```python
from build123d import *

# Parameters (mm, degrees)
SKETCH1_W                                            = 106.5
SKETCH1_H                                            = 26
BOSS_EXTRUDE1_DEPTH                                  = 8
CUT_EXTRUDE1_START                                   = -26
CUT_EXTRUDE1_OUTLINE_W                               = 6
CUT_EXTRUDE1_OUTLINE_H                               = 6.5
CUT_EXTRUDE1_OUTLINE_W_2                             = 0.5
CUT_EXTRUDE1_OUTLINE_H_2                             = 7.5
CUT_EXTRUDE1_DEPTH                                   = 26
FILLET1_R                                            = 0.5
CSK_FOR_M1_6_COUNTERSUNK_FLAT_HEAD_SCREW_D           = 1.8
CSK_FOR_M1_6_COUNTERSUNK_FLAT_HEAD_SCREW_DEPTH       = 15
CSK_FOR_M1_6_COUNTERSUNK_FLAT_HEAD_SCREW_CSINK_D     = 3.6
CSK_FOR_M1_6_COUNTERSUNK_FLAT_HEAD_SCREW_CSINK_ANGLE = 90
CSK_FOR_M1_6_COUNTERSUNK_FLAT_HEAD_SCREW_TIP         = 0.540774557
SKETCH14_W                                           = 97
SKETCH14_H                                           = 24
CUT_EXTRUDE7_DEPTH                                   = 110.919288571
SKETCH14_3_W                                         = 97
SKETCH14_3_H                                         = 24
BOSS_EXTRUDE3_DEPTH                                  = 1
SKETCH18_W                                           = 97
SKETCH18_H                                           = 24
CUT_EXTRUDE8_DEPTH                                   = 10
SKETCH20_W                                           = 97
SKETCH20_H                                           = 24
SKETCH20_W_2                                         = 93
SKETCH20_H_2                                         = 20
BOSS_EXTRUDE4_DEPTH                                  = 8
SKETCH20_2_W                                         = 97
SKETCH20_2_H                                         = 24
SKETCH20_2_W_2                                       = 93
SKETCH20_2_H_2                                       = 20
CUT_EXTRUDE9_DEPTH                                   = 1.5


# Read off the part's stored shape, not the designer's step: Cut-Extrude1
with BuildPart() as part:
    # Sketch1 → Boss-Extrude1 (new body)
    with BuildSketch(Plane(origin=(0, 0, 0), x_dir=(1, 0, 0), z_dir=(0, 1, 0))):
        with Locations((53.25, -13)):
            Rectangle(SKETCH1_W, SKETCH1_H)
    extrude(amount=BOSS_EXTRUDE1_DEPTH)

    # Cut-Extrude1 outline → Cut-Extrude1 (cut)
    with BuildSketch(Plane.XY.offset(26).offset(CUT_EXTRUDE1_START)):
        with Locations((3, 4.75)):
            Rectangle(CUT_EXTRUDE1_OUTLINE_W, CUT_EXTRUDE1_OUTLINE_H)
        with Locations((106.25, 4.25)):
            Rectangle(CUT_EXTRUDE1_OUTLINE_W_2, CUT_EXTRUDE1_OUTLINE_H_2)
    extrude(amount=CUT_EXTRUDE1_DEPTH, mode=Mode.SUBTRACT)

    # Fillet1
    fillet1_edges = [part.edges().sort_by_distance(p)[0] for p in [
        (106, 8, 13),
        (0, 1.5, 13),
        (6, 8, 13),
    ]]
    fillet(fillet1_edges, radius=FILLET1_R)

    # CSK for M1.6 Countersunk Flat Head Screw1
    with Locations(Plane(origin=(3, 1.5, 13), x_dir=(1, 0, 0), z_dir=(0, 1, 0))):
        with Locations((0, 0)):
            CounterSinkHole(CSK_FOR_M1_6_COUNTERSUNK_FLAT_HEAD_SCREW_D / 2, CSK_FOR_M1_6_COUNTERSUNK_FLAT_HEAD_SCREW_CSINK_D / 2, depth=CSK_FOR_M1_6_COUNTERSUNK_FLAT_HEAD_SCREW_DEPTH, counter_sink_angle=CSK_FOR_M1_6_COUNTERSUNK_FLAT_HEAD_SCREW_CSINK_ANGLE)
            with Locations((0, 0, -(CSK_FOR_M1_6_COUNTERSUNK_FLAT_HEAD_SCREW_DEPTH + CSK_FOR_M1_6_COUNTERSUNK_FLAT_HEAD_SCREW_TIP / 2))):  # 118° drill point
                Cone(0, CSK_FOR_M1_6_COUNTERSUNK_FLAT_HEAD_SCREW_D / 2, CSK_FOR_M1_6_COUNTERSUNK_FLAT_HEAD_SCREW_TIP, mode=Mode.SUBTRACT)

    # Sketch14 → Cut-Extrude7 (cut, through all)
    with BuildSketch(Plane(origin=(0, 8, 0), x_dir=(1, 0, 0), z_dir=(0, 1, 0))):
        with Locations((56, -13)):
            Rectangle(SKETCH14_W, SKETCH14_H)
    extrude(amount=-CUT_EXTRUDE7_DEPTH, mode=Mode.SUBTRACT)

    # Sketch14<3> → Boss-Extrude3 (add)
    with BuildSketch(Plane(origin=(0, 8, 0), x_dir=(1, 0, 0), z_dir=(0, 1, 0))):
        with Locations((56, -13)):
            Rectangle(SKETCH14_3_W, SKETCH14_3_H)
    extrude(amount=-BOSS_EXTRUDE3_DEPTH)

    # Sketch18 → Cut-Extrude8 (cut)
    with BuildSketch(Plane(origin=(0, 0, 0), x_dir=(1, 0, 0), z_dir=(0, 1, 0))):
        with Locations((56, -13)):
            Rectangle(SKETCH18_W, SKETCH18_H)
    extrude(amount=CUT_EXTRUDE8_DEPTH, mode=Mode.SUBTRACT)

    # Sketch20 → Boss-Extrude4 (add)
    with BuildSketch(Plane(origin=(0, 8, 0), x_dir=(1, 0, 0), z_dir=(0, 1, 0))):
        with Locations((56, -13)):
            Rectangle(SKETCH20_W, SKETCH20_H)
        with Locations((56, -13)):
            Rectangle(SKETCH20_W_2, SKETCH20_H_2, mode=Mode.SUBTRACT)
    extrude(amount=-BOSS_EXTRUDE4_DEPTH)

    # Sketch20<2> → Cut-Extrude9 (cut)
    with BuildSketch(Plane(origin=(0, 8, 0), x_dir=(1, 0, 0), z_dir=(0, 1, 0))):
        with Locations((56, -13)):
            Rectangle(SKETCH20_2_W, SKETCH20_2_H)
        with Locations((56, -13)):
            Rectangle(SKETCH20_2_W_2, SKETCH20_2_H_2, mode=Mode.SUBTRACT)
    extrude(amount=-CUT_EXTRUDE9_DEPTH, mode=Mode.SUBTRACT)


solid = part.part
```
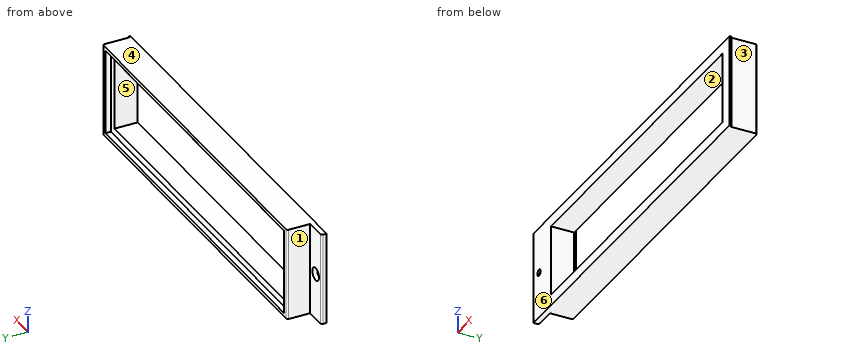
Geometry check sheet. Reference: the model listing, model coordinates, mm. Face numbers are marked on the shaded views. A direction names the side the tool comes from. Give positions to 0.01 mm unless a question says otherwise; leave off trailing zeros. Loops run counter-clockwise (first coordinate to the right, second up) from the corner with the lowest first, then second, coordinate; pieces in that order, holes last. Notation, with made-up numbers: M 5.5,75 L 63.5,75 A17 cw 63.5,88 Z; hole C 37.25,28 d8. An arc over 180 degrees is marked long. Write item = value, one per line.
(1) Sectioned sample at C-C, the plane y = 2.5. Record the cut outline in (x, z), plus the area to 3 significant figures.
Answer below:
outline = M 6,0 L 106,0 L 106,26 L 6,26 Z; hole M 9.5,3 L 102.5,3 L 102.5,23 L 9.5,23 Z
area = 740 mm2
(2) Gauge pin test, flat ends, axial feed: pin 1 Ø1.2 at (y, z) = (7.5, 11) entering from +X; pin 2 Ø0.6 at (x, z) = (106, 13.5) entering from +Y; pin 3 Ø12 at (x, z) = (56, 18.5) entering from +Y. Record the tip position at first contact, or that the pin passes through.
Answer below:
pin_1 = 106
pin_2 = 7.96
pin_3 = 6.5
(3) Sectioned sample at B-B, the plane z = 13. Record the cut outline in (x, y), plus the area to 3 significant figures.
Answer below:
outline = M 0,0 L 2.1,0 L 2.1,0.6 L 1.2,1.5 L 0.5,1.5 A0.5 ccw 0,1 Z; M 3.9,0 L 9.5,0 L 9.5,6.5 L 7.5,6.5 L 7.5,8 L 6.5,8 A0.5 ccw 6,7.5 L 6,1.5 L 4.8,1.5 L 3.9,0.6 Z; M 102.5,0 L 106.5,0 L 106.5,0.5 L 106,0.5 L 106,7.5 A0.5 ccw 105.5,8 L 104.5,8 L 104.5,6.5 L 102.5,6.5 Z
area = 55.6 mm2
(4) Sectioned sample at D-D, the plane z = 17.25. Record the cut outline in (x, y).
Answer below:
outline = M 0,0 L 9.5,0 L 9.5,6.5 L 7.5,6.5 L 7.5,8 L 6.5,8 A0.5 ccw 6,7.5 L 6,1.5 L 0.5,1.5 A0.5 ccw 0,1 Z; M 102.5,0 L 106.5,0 L 106.5,0.5 L 106,0.5 L 106,7.5 A0.5 ccw 105.5,8 L 104.5,8 L 104.5,6.5 L 102.5,6.5 Z
(5) Release check for a two-part mould opening along Z. For the marked faces 4, 5 and 6 record: released by +Z, released by -Z, zero draft, split by the parting line, or undercut.
Answer below:
face_4 = released by +Z
face_5 = undercut
face_6 = zero draft
(6) Tool access check on the marked faces 1, 2 and 3. Record the directions out of +Z, -Z, +X, -X, +Y, -Y that give a thin tool (end or side, any length) a straight path to the whole face; none if there is none.
Answer below:
face_1 = +Z, -Z, -X, +Y
face_2 = +Y, -Y
face_3 = +Z, -Z, +X, +Y
(7) Sectioned sample at A-A, the plane x = 13.5. Record the cut outline in (y, z), plus the area to 3 significant figures.
Answer below:
outline = M 0,0 L 8,0 L 8,1 L 6.5,1 L 6.5,3 L 0,3 Z; M 0,23 L 6.5,23 L 6.5,25 L 8,25 L 8,26 L 0,26 Z
area = 42.0 mm2
(8) Material ranges on line 1 (X direction, y = 0.2, z = 13); line 2 (Z direction, x = 74, y = 1.25); line 3 (Z direction, x = 3, y = 0.3), recorded low to high. Write a range as [from, to].
Answer below:
line_1 = [0, 2.1], [3.9, 9.5], [102.5, 106.5]
line_2 = [0, 3], [23, 26]
line_3 = [0, 12.1], [13.9, 26]
